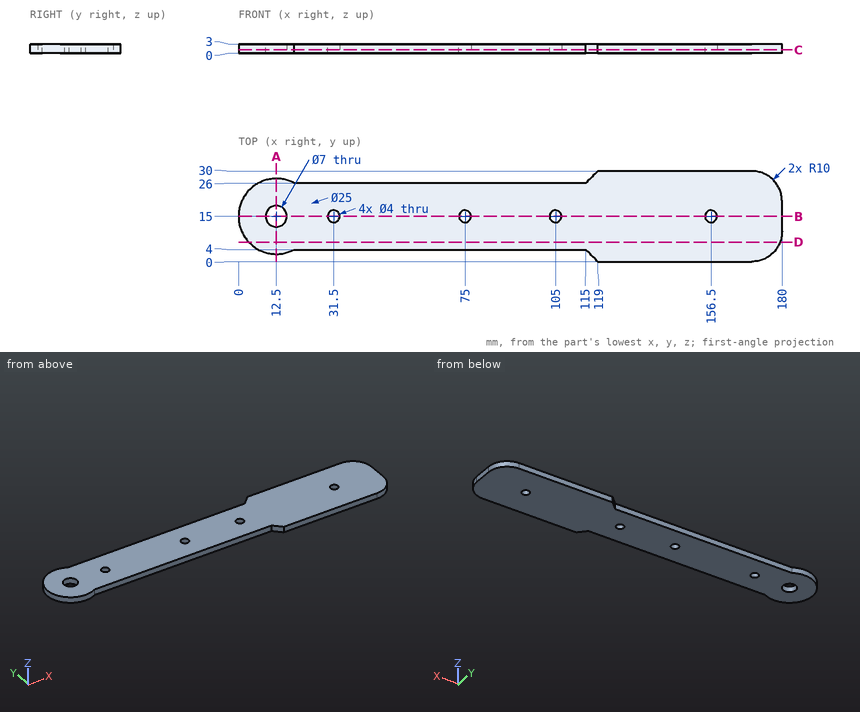
Check sheet for the drawn part. Datum: minimum x, y, z corner. Units: mm. Round coordinates to 2 decimals unless told otherwise and drop trailing zeros. Order: outer loops, then holes, each group sorted by start corner. A loop starts at its lowest first (then second) coordinate and runs counter-clockwise, first axis right, second up.
1) Scan lines: line 1 (Y direction, x = 75, z = 2.25); line 2 (Y direction, x = 22, z = 2.4); line 3 (Y direction, x = 156.5, z = 0.7). Record each from-to range of solid material in increasing order.
2) Section check B-B (y = 15). Record the boundary of the cut face in (x, z), and give its area (3 significant figures).
3) Section check A-A (x = 12.5). Record the boundary of the cut face in (y, z).
4) Section check D-D (y = 6.5). Record the boundary of the cut face in (x, z) (1 decimal).
5) Section check C-C (z = 1.05). Give the number of separate pieces and of enclosed holes in the cut face, and give its area (3 significant figures).
6) Go/stop test with flat-tipped pins: pin 1 Ø3.5 at (x, y) = (31.5, 15) entering from -Z; pin 2 Ø1.5 at (x, y) = (54, 5.5) entering from -Z; pin 3 Ø1.5 at (x, z) = (65.5, 1) entering from +Y; pin 4 Ø1 at (y, z) = (19.5, 1.5) entering from -X. Record where each tip stops, or that it passes through.
Result:
1. line 1: y = 4 to 13, 17 to 26
1. line 2: y = 4 to 26
1. line 3: y = 0 to 13, 17 to 30
2. outline: (0, 0) - (9, 0) - (9, 3) - (0, 3) - close; (16, 0) - (29.5, 0) - (29.5, 3) - (16, 3) - close; (33.5, 0) - (73, 0) - (73, 3) - (33.5, 3) - close; (77, 0) - (103, 0) - (103, 3) - (77, 3) - close; (107, 0) - (154.5, 0) - (154.5, 3) - (107, 3) - close; (158.5, 0) - (180, 0) - (180, 3) - (158.5, 3) - close
2. area: 471 mm2
3. outline: (2.5, 0) - (11.5, 0) - (11.5, 3) - (2.5, 3) - close; (18.5, 0) - (27.5, 0) - (27.5, 3) - (18.5, 3) - close
4. outline: (3.3, 0) - (179.4, 0) - (179.4, 3) - (3.3, 3) - close
5. separate pieces: 1
5. enclosed holes: 5
5. area: 4,310 mm2
6. pin 1: passes through
6. pin 2: stops at z = 0
6. pin 3: stops at y = 26
6. pin 4: stops at x = 0.66
